Could you check a few things on this model? Use its own coordinates, in mm. A direction names the side the tool comes from. Give positions to 0.01 mm unless a question says otherwise; leave off trailing zeros. Write each loop counter-clockwise with the first axis right and the second up, starting at its lowest first coordinate (ties: lowest second). Pieces come first, ordered by that corner, then holes. Notation, with made-up numbers: (56, 87) - (60, 87) arc R8 ccw to (60, 98) - close; hole circle Ø11 at (-1.5, -10). An arc over 180 degrees is marked (long way). Answer in a Markdown table with one row per item.
from build123d import *

# Parameters (mm, degrees)
SKIZZE1_R                                            = 92.5
AUFSATZ_LINEAR_AUSTRAGEN1_DEPTH                      = 10
STIRNSENKUNG_F_R_M4_ZYLINDERSCHRAUBE_MIT_D           = 4.5
STIRNSENKUNG_F_R_M4_ZYLINDERSCHRAUBE_MIT_CBORE_D     = 8
STIRNSENKUNG_F_R_M4_ZYLINDERSCHRAUBE_MIT_CBORE_DEPTH = 4.4
SKIZZE10_OUTSIDE_W                                   = 239.364
SKIZZE10_OUTSIDE_H                                   = 239.364
SCHNITT_LINEAR_AUSTRAGEN1_DEPTH                      = 132.196417634
VERRUNDUNG2_R                                        = 10
VERRUNDUNG3_R                                        = 75
SCHNITT_LINEAR_AUSTRAGEN2_REACH                      = 132.221
SKIZZE14_R                                           = 2.15
SKIZZE15_R                                           = 4
SCHNITT_LINEAR_AUSTRAGEN3_DEPTH                      = 4.4
M3_GEWINDEBOHRUNG1_D                                 = 2.5
M3_GEWINDEBOHRUNG1_DEPTH                             = 8.5
M3_GEWINDEBOHRUNG1_TIP                               = 0.751075774


with BuildPart() as part:
    # Skizze1 → Aufsatz-Linear austragen1 (new body)
    with BuildSketch(Plane.XY):
        Circle(SKIZZE1_R)
    extrude(amount=AUFSATZ_LINEAR_AUSTRAGEN1_DEPTH)

    # Stirnsenkung für M4 Zylinderschraube mit Innensechskant1 (through all)
    with Locations(Plane(origin=(-81.25, -15.25, 10), x_dir=(1, 0, 0), z_dir=(0, 0, 1))):
        with Locations((0, 0), (22.5, 0), (97.418112592, 73.753992472), (108.668112592, 93.239564057), (123.831887408, -28.003992472), (135.081887408, -47.489564057), (120.79663337, -42.746778265), (111.70336663, 78.496778265), (11.25, 10)):
            CounterBoreHole(STIRNSENKUNG_F_R_M4_ZYLINDERSCHRAUBE_MIT_D / 2, STIRNSENKUNG_F_R_M4_ZYLINDERSCHRAUBE_MIT_CBORE_D / 2, STIRNSENKUNG_F_R_M4_ZYLINDERSCHRAUBE_MIT_CBORE_DEPTH)

    # Skizze10 outside → Schnitt-Linear austragen1 (cut, through all)
    with BuildSketch(Plane(origin=(0, 0, 0), x_dir=(-1, 0, 0), z_dir=(0, 0, -1))):
        Rectangle(SKIZZE10_OUTSIDE_W, SKIZZE10_OUTSIDE_H)
        with BuildLine():
            Line((86.602540378, -32.5), (18.763883749, -32.5))
            Line((18.763883749, -32.5), (-15.155444566, -91.25))
            ThreePointArc((-15.155444566, -91.25), (-48.569408387, -78.722694116), (-74.754788955, -54.479092579))
            Line((-74.754788955, -54.479092579), (-40.414518843, 5))
            Line((-40.414518843, 5), (-71.447095812, 58.75))
            ThreePointArc((-71.447095812, 58.75), (-43.891148765, 81.423688568), (-9.802883671, 91.979092579))
            Line((-9.802883671, 91.979092579), (21.650635095, 37.5))
            Line((21.650635095, 37.5), (84.557672626, 37.5))
            ThreePointArc((84.557672626, 37.5), (92.460557153, 2.700994452), (86.602540378, -32.5))
        make_face(mode=Mode.SUBTRACT)
    extrude(amount=-SCHNITT_LINEAR_AUSTRAGEN1_DEPTH, mode=Mode.SUBTRACT)

    # Verrundung2
    verrundung2_edges = [part.edges().sort_by_distance(p)[0] for p in [
        (15.155444566, -91.25, 5),
        (74.754788955, -54.479092579, 5),
        (71.447095812, 58.75, 5),
        (9.802883671, 91.979092579, 5),
        (-84.557672626, 37.5, 5),
        (-86.602540378, -32.5, 5),
    ]]
    fillet(verrundung2_edges, radius=VERRUNDUNG2_R)

    # Verrundung3
    verrundung3_edges = [part.edges().sort_by_distance(p)[0] for p in [
        (-18.763883749, -32.5, 5),
        (40.414518843, 5, 5),
        (-21.650635095, 37.5, 5),
    ]]
    fillet(verrundung3_edges, radius=VERRUNDUNG3_R)

    # Skizze14 → Schnitt-Linear austragen2 (cut, up to next)
    with BuildSketch(Plane.XY.offset(10), mode=Mode.PRIVATE) as schnitt_linear_austragen2_sk1:
        with Locations((-17.5, 30)):
            Circle(SKIZZE14_R)
    schnitt_linear_austragen2_tool1 = extrude(schnitt_linear_austragen2_sk1.sketch, amount=-SCHNITT_LINEAR_AUSTRAGEN2_REACH, mode=Mode.PRIVATE) & part.part
    # Skizze14 → Schnitt-Linear austragen2 (cut, up to next)
    with BuildSketch(Plane.XY.offset(10), mode=Mode.PRIVATE) as schnitt_linear_austragen2_sk2:
        with Locations((-17.5, -30)):
            Circle(SKIZZE14_R)
    schnitt_linear_austragen2_tool2 = extrude(schnitt_linear_austragen2_sk2.sketch, amount=-SCHNITT_LINEAR_AUSTRAGEN2_REACH, mode=Mode.PRIVATE) & part.part
    add(schnitt_linear_austragen2_tool1.solids().sort_by_distance((-17.5, 30, 10))[0], mode=Mode.SUBTRACT)
    add(schnitt_linear_austragen2_tool2.solids().sort_by_distance((-17.5, -30, 10))[0], mode=Mode.SUBTRACT)

    # Skizze15 → Schnitt-Linear austragen3 (cut)
    with BuildSketch(Plane(origin=(0, 0, 0), x_dir=(-1, 0, 0), z_dir=(0, 0, -1))):
        with Locations((17.5, 30)):
            Circle(SKIZZE15_R)
        with Locations((17.5, -30)):
            Circle(SKIZZE15_R)
    extrude(amount=-SCHNITT_LINEAR_AUSTRAGEN3_DEPTH, mode=Mode.SUBTRACT)

    # M3 Gewindebohrung1
    with Locations(Plane(origin=(0, 0, 0), x_dir=(-1, 0, 0), z_dir=(0, 0, -1))):
        with Locations((82.5, -4.5), (82.5, 14.5), (-45.147114317, -69.197095812), (-28.692631645, -78.697095812), (-37.352885683, 73.697095812), (-53.807368355, 64.197095812), (0, 0)):
            Hole(M3_GEWINDEBOHRUNG1_D / 2, depth=M3_GEWINDEBOHRUNG1_DEPTH)
            with Locations((0, 0, -(M3_GEWINDEBOHRUNG1_DEPTH + M3_GEWINDEBOHRUNG1_TIP / 2))):  # 118° drill point
                Cone(0, M3_GEWINDEBOHRUNG1_D / 2, M3_GEWINDEBOHRUNG1_TIP, mode=Mode.SUBTRACT)


solid = part.part
1) Imagine slicing it at A-A (x = -17.5). List the corners of the cut face in (y, z) for me, then the cut area to 3 significant figures.
Check values:
| item | result |
|---|---|
| outline | (-47.18, 0) - (-34, 0) - (-34, 4.4) - (-32.15, 4.4) - (-32.15, 10) - (-47.18, 10) - close; (-27.85, 4.4) - (-26, 4.4) - (-26, 0) - (26, 0) - (26, 4.4) - (27.85, 4.4) - (27.85, 10) - (-27.85, 10) - close; (32.15, 4.4) - (34, 4.4) - (34, 0) - (54.42, 0) - (54.42, 10) - (32.15, 10) - close |
| area | 897 mm2 |
2) Imagine slicing it at B-B (y = -30). List the corners of the cut face in (x, z) for me, then the cut area to 3 significant figures.
Check values:
| item | result |
|---|---|
| outline | (-85.99, 0) - (-21.5, 0) - (-21.5, 4.4) - (-19.65, 4.4) - (-19.65, 10) - (-85.99, 10) - close; (-15.35, 4.4) - (-13.5, 4.4) - (-13.5, 0) - (60.68, 0) - (60.68, 10) - (-15.35, 10) - close |
| area | 1,410 mm2 |
3) Imagine slicing it at C-C (y = -74). List the corners of the cut face in (x, z) for me, then the cut area to 3 significant figures.
Check values:
| item | result |
|---|---|
| outline | (5.2, 0) - (55.5, 0) - (55.5, 10) - (5.2, 10) - close |
| area | 503 mm2 |
4) Will these pins go through, and if not, where does the flat tip stop? P1, Ø6, axis at y = 8, z = 2.5, coming from the -X side; P2, Ø2.5, axis at x = -60, y = -13.5, coming from the +Z side; P3, Ø3.5, axis at x = 42.58, y = -43.25, coming from the -Z side; P4, Ø3, axis at x = -67, z = 6, coming from the -Y side.
Check values:
| item | result |
|---|---|
| P1 | stops at x = -92.36 |
| P2 | stops at z = 5.6 |
| P3 | passes through |
| P4 | stops at y = -32.5 |
5) On a 3-axis mill with a long thin cutter (end or side, diameter ignored), from which of +Z, -Z, +X, -X, +Y, -Y can I reach the whole of each face in a straight line? I mean faces 1 (the face through (-71, -32.5, 5)), 2 (the face through (29.59, 59.34, 7.83)), 3 (the face through (-16.979, -26.034, 2.169)), 4 (the face through (66.8, -40.7, 4.9)). Say none if no direction works.
Check values:
| item | result |
|---|---|
| face 1 | +Z, -Z, -X, -Y |
| face 2 | +Z |
| face 3 | -Z |
| face 4 | +Z, -Z, +X |
6) If I drill on line 1 (Y direction, x = -17.5, z = 7.15); line 2 (Y direction, x = -70, z = 2.55); line 3 (Y direction, x = 59.5, z = 7.5), over which ranges is the centre line in solid material (lowest first)?
Check values:
| item | result |
|---|---|
| line 1 | y = -47.18 to -32.15, -27.85 to 27.85, 32.15 to 54.42 |
| line 2 | y = -32.5 to -7.5, -3 to 37.5 |
| line 3 | y = -70.82 to -27.66, 37.66 to 70.82 |
7) We'd pull the mould along Y, two halves only. Please class faces 5 (the face through (48.43, -78.81, 4.93)), 6 (the face through (46.277, -44.786, 7.831)), 7 (the face through (-19, -32, 4.4)), 8 (the face through (-83.63, 35.61, 5.07)): +Y half, -Y half, draft (parallel to the pull), parting line (faces both ways), or undercut.
Check values:
| item | result |
|---|---|
| face 5 | -Y half |
| face 6 | undercut |
| face 7 | undercut |
| face 8 | +Y half |
